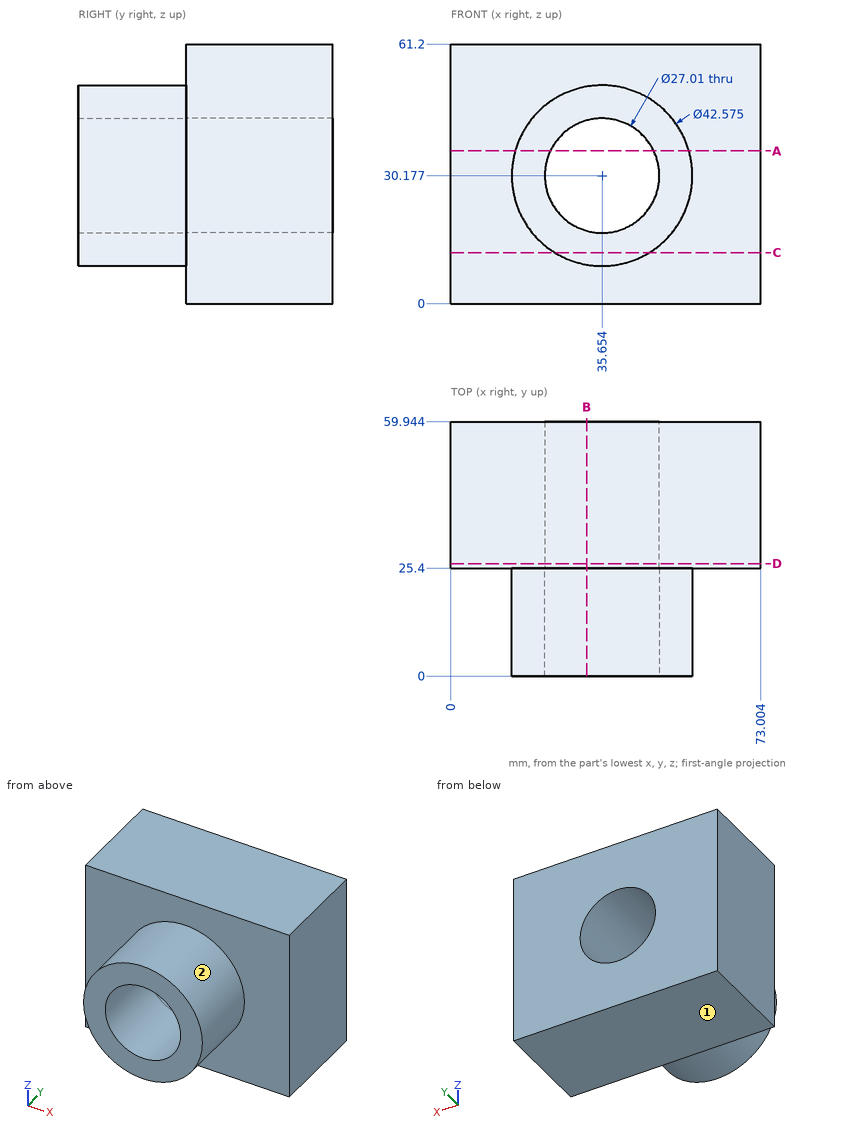
Answer from the drawing. Dimensions are ordinates in mm from the lowest x, y and z of the part. A direction names the side the tool comes from. Round coordinates to 2 decimals unless told otherwise and drop trailing zeros. Write each loop counter-clockwise with the first axis right and the second up, starting at its lowest first coordinate (ties: lowest second). Pieces come first, ordered by that corner, then holes. Notation, with made-up numbers: (74.5, 89.5) - (110.5, 89.5) arc R27 cw to (110.5, 123.5) - close; hole circle Ø2 at (3.5, 79). An arc over 180 degrees is marked (long way). Use a Markdown table: item, result.
(1) Which of the six approach directions +Z, -Z, +X, -X, +Y, -Y give full straight-line access (tool end or side, diameter ignored) to the marked faces 1 and 2?
Reported:
| item | result |
|---|---|
| face 1 | -Z, +X, -X, +Y, -Y |
| face 2 | -Y |
(2) Straight lines are drawn through the part: line 1 along X through (y, z) = (18.5, 30.5) (1 decimal); line 2 along Y through (x, z) = (16, 14); line 3 along Z through (x, y) = (28.5, 9.5) (1 decimal). For each, find the intervals that lie inside material, in ascending order. Write a range as [from, to].
Reported:
| item | result |
|---|---|
| line 1 | [14.4, 22.2], [49.2, 56.9] |
| line 2 | [25.4, 59.94] |
| line 3 | [10.1, 18.7], [41.6, 50.2] |
(3) The part is cut by section B-B (x = 32). Write down the section's boundary in (y, z) (1 decimal), then the cut area to 3 significant figures.
Reported:
| item | result |
|---|---|
| outline | (0, 9.2) - (25.4, 9.2) - (25.4, 0) - (59.9, 0) - (59.9, 17.2) - (0, 17.2) - close; (0, 43.2) - (59.9, 43.2) - (59.9, 61.2) - (25.4, 61.2) - (25.4, 51.1) - (0, 51.1) - close |
| area | 1,620 mm2 |
(4) The part is cut by section A-A (z = 36). Write down the section's boundary in (x, y) (1 decimal).
Reported:
| item | result |
|---|---|
| outline | (0, 25.4) - (15.2, 25.4) - (15.2, 0) - (23.5, 0) - (23.5, 59.9) - (0, 59.9) - close; (47.8, 0) - (56.1, 0) - (56.1, 25.4) - (73, 25.4) - (73, 59.9) - (47.8, 59.9) - close |
(5) The part is cut by section C-C (z = 12). Write down the section's boundary in (x, y) (1 decimal).
Reported:
| item | result |
|---|---|
| outline | (0, 25.4) - (24.6, 25.4) - (24.6, 0) - (46.7, 0) - (46.7, 25.4) - (73, 25.4) - (73, 59.9) - (0, 59.9) - close |
(6) The part is cut by section D-D (y = 26.5). Write down the section's boundary in (x, z) (1 decimal).
Reported:
| item | result |
|---|---|
| outline | (0, 0) - (73, 0) - (73, 61.2) - (0, 61.2) - close; hole circle Ø27 at (35.7, 30.2) |
(7) This flat-tipped pin is pushed along its axis until it touches: pin 1 Ø1.5 at (y, z) = (13.5, 36.5) entering from +X. Where does it stop, or does it pass through?
Reported:
| item | result |
|---|---|
| pin 1 | x = 56.2 |
